Design review of the part shown in the three views and the two pictorial views. Dimensions are in mm from the part's minimum x, y and z. A direction names the side the tool comes from. Round coordinates to 2 decimals unless told otherwise and drop trailing zeros. Loops run counter-clockwise (first coordinate to the right, second up) from the corner with the lowest first, then second, coordinate; pieces in that order, holes last. Notation, with made-up numbers: M 87.25,-9.5 L 93.25,-9.5 A15 cw 93.25,-2.5 Z; hole C -8,4.5 d11. An arc over 180 degrees is marked long. One line per question, with ' | ' between items.
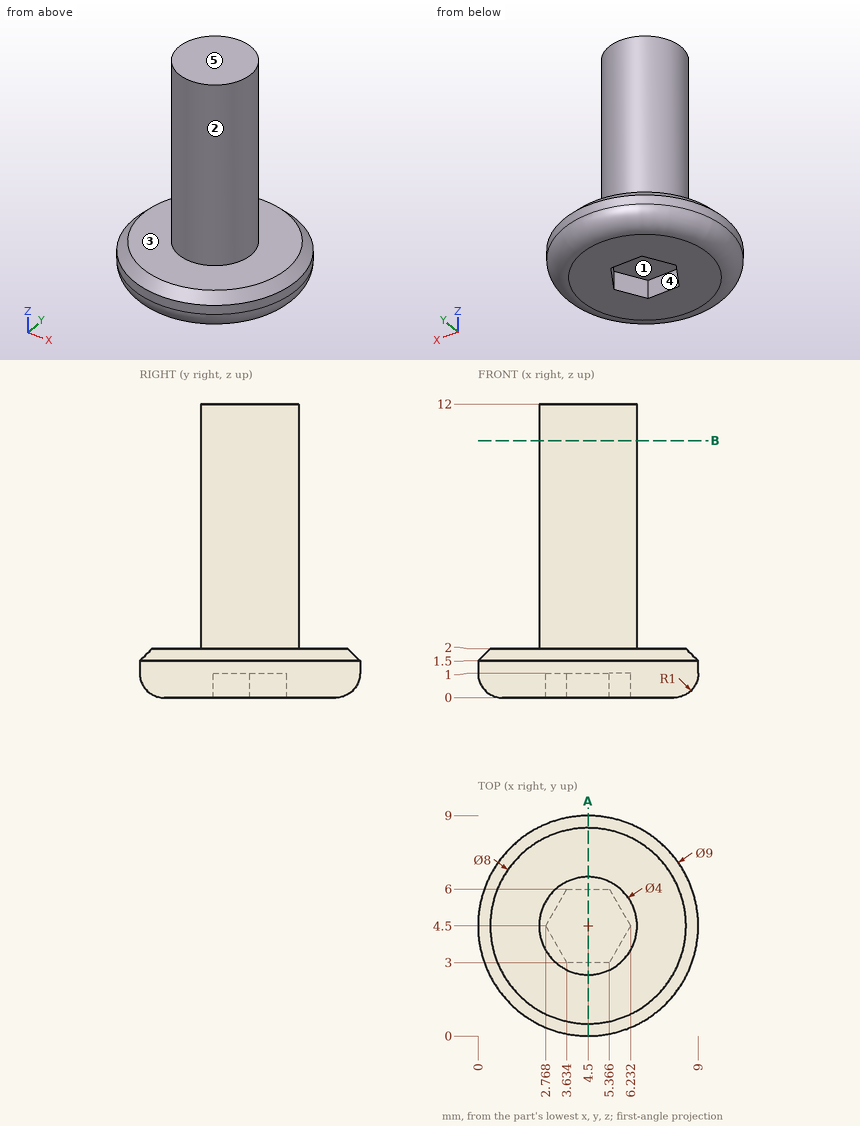
1) For line 1 (Z direction, x = 6.75, y = 5.75); line 2 (Y direction, x = 3.5, z = 10.75), list the stretches that pass through material, from the lowest coordinate up.
Output values:
line 1: z = 0 to 2 | line 2: y = 2.77 to 6.23
2) Add section B-B on z = 10.5. State the section outline as (x, y) points.
Output values:
outline: C 4.5,4.5 d4
3) Add section A-A on x = 4.5. State the section outline as (y, z) points.
Output values:
outline: M 0,1 A1 ccw 1,0 L 3,0 L 3,1 L 6,1 L 6,0 L 8,0 A1 ccw 9,1 L 9,1.5 L 8.5,2 L 6.5,2 L 6.5,12 L 2.5,12 L 2.5,2 L 0.5,2 L 0,1.5 Z
4) Machinability: for the marked faces 4 and 5, which of the approach directions +Z, -Z, +X, -X, +Y, -Y give a long, thin tool a straight path to every point of the face, cutting with its end or side? Answer none if there is none.
Output values:
face 4: -Z | face 5: +Z, +X, -X, +Y, -Y
5) Insertion check: P1, Ø0.8, axis at x = 4.5, z = 0.5, coming from the +Y side (3 decimals); P2, Ø5, axis at x = 3.5, z = 8, coming from the -Y side; P3, Ø0.5, axis at x = 5, z = 0.5, coming from the -Y side (3 decimals). Each pin has a flat end and moves straight along its axis. Give the tip position at first contact, or say it passes through.
Output values:
P1: stops at y = 8.995 | P2: stops at y = 2.5 | P3: stops at y = 0.055
6) Mouldability with a two-part tool opening along Y and no side actions: class the marked faces 1, 2 and 3 as +Y half, -Y half, draft (parallel to the pull), parting line (faces both ways), or undercut.
Output values:
face 1: undercut | face 2: parting line | face 3: draft
